from build123d import *

# Parameters (mm, degrees)
DODANIE_WYCI_GNI_CIE2_DEPTH = 1.5
SZKIC37_R                   = 1.85
DODANIE_WYCI_GNI_CIE3_DEPTH = 1.5
SZKIC38_R                   = 3.85
DODANIE_WYCI_GNI_CIE4_DEPTH = 1.7
ZAOKR_GLENIE1_R             = 2
SZKIC39_R                   = 2.35
DODANIE_WYCI_GNI_CIE5_DEPTH = 10
SZKIC40_W                   = 20
SZKIC40_H                   = 1
DODANIE_WYCI_GNI_CIE6_DEPTH = 4
SFAZOWANIE1_SIZE            = 1


# Some blends are built 0.0001 mm under size
with BuildPart() as part:
    # Szkic35 → Dodanie-wyciągnięcie2 (new body)
    with BuildSketch(Plane.XY):
        with BuildLine():
            Line((-15, -11.5), (-15, 11.5))
            ThreePointArc((-15, 11.5), (0, 26.5), (15, 11.5))
            Line((15, 11.5), (15, -11.5))
            ThreePointArc((15, -11.5), (0, -26.5), (-15, -11.5))
        make_face()
    extrude(amount=DODANIE_WYCI_GNI_CIE2_DEPTH)

    # Szkic37 → Dodanie-wyciągnięcie3 (add)
    with BuildSketch(Plane(origin=(0, 0, 0), x_dir=(-1, 0, 0), z_dir=(0, 0, -1))):
        with Locations((0, 12.5)):
            Circle(SZKIC37_R)
        with Locations((0, -12.5)):
            Circle(SZKIC37_R)
    extrude(amount=DODANIE_WYCI_GNI_CIE3_DEPTH)

    # Szkic38 → Dodanie-wyciągnięcie4 (add)
    with BuildSketch(Plane(origin=(0, 0, -1.5), x_dir=(-1, 0, 0), z_dir=(0, 0, -1))):
        with Locations((0, 12.5)):
            Circle(SZKIC38_R)
        with Locations((0, -12.5)):
            Circle(SZKIC38_R)
    extrude(amount=DODANIE_WYCI_GNI_CIE4_DEPTH)

    # Zaokrąglenie1
    # the kernel refuses this fillet: 2 mm, written as the material it takes off along each edge
    with BuildSketch(Plane(origin=(0, 12.5, -3.2), x_dir=(-1, 0, 0), z_dir=(0, -1, 0))) as zaokr_glenie1_piece_1:
        with BuildLine():
            CenterArc((1.872628007, -2), ZAOKR_GLENIE1_R, 8.626926559, 81.373073441)
            Line((1.872628007, 0), (1.872628007, 0.04))
            Line((1.872628007, 0.04), (3.85, 0.04))
            Line((3.85, 0.04), (3.89, 0))
            ThreePointArc((3.89, 0), (3.89, -0.85), (3.88954744, -1.694))
            Line((3.88954744, -1.694), (3.85, -1.7))
        make_face()
    revolve(axis=Axis((0, 12.5, -3.2), (0, 0, -1)), mode=Mode.SUBTRACT)
    with BuildSketch(Plane(origin=(0, -12.5, -3.2), x_dir=(-1, 0, 0), z_dir=(0, -1, 0))) as zaokr_glenie1_piece_2:
        with BuildLine():
            CenterArc((1.872628007, -2), ZAOKR_GLENIE1_R, 8.626926559, 81.373073441)
            Line((1.872628007, 0), (1.872628007, 0.04))
            Line((1.872628007, 0.04), (3.85, 0.04))
            Line((3.85, 0.04), (3.89, 0))
            ThreePointArc((3.89, 0), (3.89, -0.85), (3.88954744, -1.694))
            Line((3.88954744, -1.694), (3.85, -1.7))
        make_face()
    revolve(axis=Axis((0, -12.5, -3.2), (0, 0, -1)), mode=Mode.SUBTRACT)

    # Szkic39 → Dodanie-wyciągnięcie5 (add)
    with BuildSketch(Plane.XY.offset(1.5)):
        with Locations(Location((0, 0, 0), (0, 0, 180))):
            Circle(SZKIC39_R)
    extrude(amount=DODANIE_WYCI_GNI_CIE5_DEPTH)

    # Szkic40 → Dodanie-wyciągnięcie6 (add)
    with BuildSketch(Plane.XY.offset(1.5)):
        with Locations((0, 10.5)):
            Rectangle(SZKIC40_W, SZKIC40_H)
        with Locations((0, -10.5)):
            Rectangle(SZKIC40_W, SZKIC40_H)
    extrude(amount=DODANIE_WYCI_GNI_CIE6_DEPTH)

    # Sfazowanie1
    sfazowanie1_edges = [part.edges().sort_by_distance(p)[0] for p in [
        (0, 11, 5.5),
        (0, -11, 5.5),
    ]]
    chamfer(sfazowanie1_edges, length=SFAZOWANIE1_SIZE - 0.0001)  # a hair under: the kernel refuses the full size


solid = part.part
Work out the finished part from the listing and answer in its coordinate system (mm). A direction names the side the tool comes from. Give positions to 0.01 mm unless a question says otherwise; leave off trailing zeros. Order: outer loops, then holes, each group sorted by start corner. A loop starts at its lowest first (then second) coordinate and runs counter-clockwise, first axis right, second up. Notation, with made-up numbers: M 7,22.5 L 33,22.5 A16 ccw 33,48.5 Z; hole C -10.75,-39 d8. An arc over 180 degrees is marked long. Return JSON: item names as keys, results as strings.
Q1. Find the intervals of material crossed by line 1 along Y through (x, z) = (6.5, 4.5); line 2 along Z through (x, y) = (-10.5, -14); line 3 along Y through (x, z) = (2.5, -2), in increasing order. Write a range as [from, to].
Answer below:
{"line 1": "y = [-11, -10], [10, 11]", "line 2": "z = [0, 1.5]", "line 3": "y = [-15.24, -9.76], [9.76, 15.24]"}
Q2. Find section C-C, the plane z = 6.5. Write down the section's boundary in (x, y), and give its area (3 significant figures).
Answer below:
{"outline": "C 0,0 d4.7", "area": "17.3 mm^2"}
Q3. Which of the six approach directions +Z, -Z, +X, -X, +Y, -Y give full straight-line access (tool end or side, diameter ignored) to faces 4 (the face through (0.509, 2.294, 6.43)), 5 (the face through (10, -10.5, 3)), 6 (the face through (-2, -12, -1.5)), 7 (the face through (-10, -10.5, 3)), 8 (the face through (0, 10, 3))?
Answer below:
{"face 4": "+Z", "face 5": "+Z, +X, +Y, -Y", "face 6": "none", "face 7": "+Z, -X, +Y, -Y", "face 8": "+Z, +X, -X"}
Q4. Find section B-B, the plane y = 0. Write down the section's boundary in (x, z).
Answer below:
{"outline": "M -15,0 L 15,0 L 15,1.5 L 2.35,1.5 L 2.35,11.5 L -2.35,11.5 L -2.35,1.5 L -15,1.5 Z"}
Q5. Each of these flat-tipped pins is pushed along its axis until it touches: pin 1 (1.1 mm diameter, centred on y = 10.5, z = 3.5, fed in from -X); pin 2 (10 mm diameter, centred on x = -7, y = -7.5, fed in from -Z); pin 3 (8 mm diameter, centred on x = 9.5, z = 1.5, fed in from +Y); pin 4 (4 mm diameter, centred on y = 11.5, z = -0.5, fed in from -X). Where does it stop, or does it pass through?
Answer below:
{"pin 1": "stops at x = -10", "pin 2": "stops at z = -2.2", "pin 3": "stops at y = 25.46", "pin 4": "stops at x = -15"}
Q6. The mould has two halves that part along Z. Classify faces 1 (the face through (0, 11, 3)), 2 (the face through (-0.1, -10.5, 5)), 3 (the face through (-2, 13, -1.5)): pulls with the +Z half, pulls with the -Z half, needs draft (parallel to the pull), parting line crosses it, or undercut.
Answer below:
{"face 1": "needs draft", "face 2": "pulls with the +Z half", "face 3": "undercut"}
